Read the model definition and answer for the solid it produces. Units are mm, in the model's axes. Face numbers are marked on the shaded views. A direction names the side the tool comes from. Coordinates: 2 decimals unless noted, no trailing zeros. Write each loop counter-clockwise with the first axis right and the second up, starting at its lowest first coordinate (ties: lowest second). Pieces come first, ordered by that corner, then holes.
1) The part is cut by section B-B (y = -22). Determine the outline of the cut face in (x, z).
2) Which of the six approach directions +Z, -Z, +X, -X, +Y, -Y give full straight-line access (tool end or side, diameter ignored) to the marked faces 1 and 2?
3) Find the intervals of material crossed by line 1 (X direction, y = -17, z = 27); line 2 (Y direction, x = 48, z = 25); line 3 (Y direction, x = -16.5, z = 15.5), in increasing order.
4) The part is cut by section C-C (x = -3.5). Determine the outline of the cut face in (y, z), then the cut area to 3 significant figures.
5) Determine the mould class of the marked faces 3, 4 and 5 for opening direction Y: +Y half, -Y half, draft (parallel to the pull), parting line (faces both ways), or undercut.
6) The part is cut by section A-A (z = 40.5). Determine the outline of the cut face in (x, y), then the cut area to 3 significant figures.
7) Each of these flat-tipped pins is pushed along its axis until it touches: pin 1 Ø17.5 at (y, z) = (0, 25.4) entering from +X; pin 2 Ø3 at (x, y) = (-6.5, -41) entering from +Z. Where does it stop, or does it pass through?
8) The part is cut by section D-D (y = 0). Determine the outline of the cut face in (x, z).
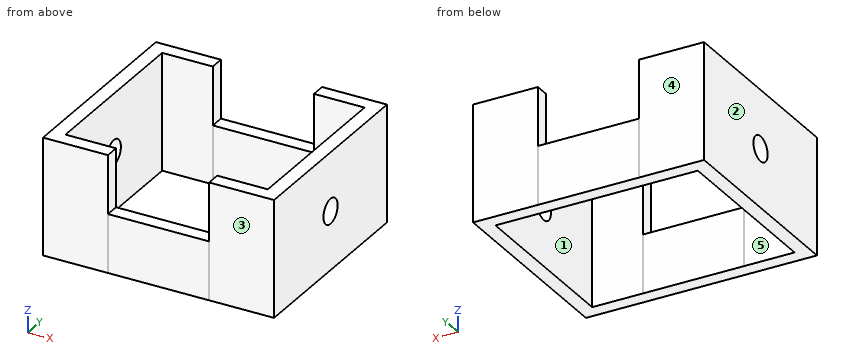
from build123d import *

# Parameters (mm, degrees)
F1_DEPTH = 50.8
F0_W     = 22.011524
F0_H     = 6.233353
F2_DEPTH = 25.4
F4_R     = 5.436112
F5_DEPTH = 50.257401


with BuildPart() as f1:
    # F0 (on Top) → F1 (new body)
    with BuildSketch(Plane.XY):
        Polygon((-50.256401, -43.438673), (-22.011524, -43.438673), (-22.011524, -37.20532), (-44.023048, -37.20532), (-44.023048, 0), (-50.256401, 0), align=None)
    extrude(amount=F1_DEPTH)

    # F0 (on Top) → F2 (join)
    with BuildSketch(Plane.XY):
        with Locations((-11.005762, -40.321996)):
            Rectangle(F0_W, F0_H)
        Polygon((-50.256401, -43.438673), (-22.011524, -43.438673), (-22.011524, -37.20532), (-44.023048, -37.20532), (-44.023048, 0), (-50.256401, 0), align=None)
    extrude(amount=F2_DEPTH)

    # F3: F1 across plane


with BuildPart() as f1_1:
    add(f1.part)
    add(f1.part.mirror(Plane.XZ))

    # F4 (on face) → F5 (cut, through all)
    with BuildSketch(Plane(origin=(-50.256401, 0, 0), x_dir=(0, -1, 0), z_dir=(-1, 0, 0))):
        with Locations((0, 25.4)):
            Circle(F4_R)
    extrude(amount=-F5_DEPTH, mode=Mode.SUBTRACT)

    # F6: F1 across plane


with BuildPart() as f1_2:
    add(f1_1.part)
    add(f1_1.part.mirror(Plane.YZ))


solid = f1_2.part
Reported:
1. outline: (-50.26, 0) - (-44.02, 0) - (-44.02, 50.8) - (-50.26, 50.8) - close; (44.02, 0) - (50.26, 0) - (50.26, 50.8) - (44.02, 50.8) - close
2. face 1: +Z, -Z
2. face 2: +Z, -Z, -X, +Y, -Y
3. line 1: x = -50.26 to -44.02, 44.02 to 50.26
3. line 2: y = -43.44 to -5.42, 5.42 to 43.44
3. line 3: y = -43.44 to -37.21, 37.21 to 43.44
4. outline: (-43.44, 0) - (-37.21, 0) - (-37.21, 25.4) - (-43.44, 25.4) - close; (37.21, 0) - (43.44, 0) - (43.44, 25.4) - (37.21, 25.4) - close
4. area: 317 mm2
5. face 3: -Y half
5. face 4: +Y half
5. face 5: undercut
6. outline: (-50.26, -43.44) - (-22.01, -43.44) - (-22.01, -37.21) - (-44.02, -37.21) - (-44.02, 37.21) - (-22.01, 37.21) - (-22.01, 43.44) - (-50.26, 43.44) - close; (22.01, -43.44) - (50.26, -43.44) - (50.26, 43.44) - (22.01, 43.44) - (22.01, 37.21) - (44.02, 37.21) - (44.02, -37.21) - (22.01, -37.21) - close
6. area: 1,630 mm2
7. pin 1: stops at x = 50.26
7. pin 2: stops at z = 25.4
8. outline: (-50.26, 0) - (-44.02, 0) - (-44.02, 19.96) - (-50.26, 19.96) - close; (-50.26, 30.84) - (-44.02, 30.84) - (-44.02, 50.8) - (-50.26, 50.8) - close; (44.02, 0) - (50.26, 0) - (50.26, 19.96) - (44.02, 19.96) - close; (44.02, 30.84) - (50.26, 30.84) - (50.26, 50.8) - (44.02, 50.8) - close
